Check sheet for the modelled part. Datum: model origin and axes. Units: mm. A direction names the side the tool comes from. Give positions to 0.01 mm unless a question says otherwise; leave off trailing zeros. Order: outer loops, then holes, each group sorted by start corner. A loop starts at its lowest first (then second) coordinate and runs counter-clockwise, first axis right, second up.
Autodesk Inventor part; units mm, degrees
ref_plane "Work Plane1" through (80, 0, 9.5) normal (0, 0, 1) x (1, 0, 0)
ref_plane "YZ Plane" through (0, 0, 0) normal (1, 0, 0) x (0, 1, 0)
ref_plane "XZ Plane" through (0, 0, 0) normal (0, 1, 0) x (-1, 0, 0)
sketch "Sketch1" plane through (0, 0, 0) normal (0, 0, 1) x (1, 0, 0)
  line L0 (0, 0) -> (115, 0)
  line L1 (115, 0) -> (115, 8.2)
  line L2 (115, 8.2) -> (-25, 8.2)
  line L3 (-25, 8.2) -> (-460, 8.2)
  line L4 (-460, 8.2) -> (-460, 0)
  line L5 (-460, 0) -> (0, 0)
  line L6 (-340, 8.2) -> (-340, 8.5)
  line L7 (-340, 8.5) -> (-390, 8.5)
  line L8 (-390, 8.5) -> (-390, 8.2)
  line L9 (15, 8.2) -> (15, 8.5)
  line L10 (15, 8.5) -> (-30, 8.5)
  line L11 (-30, 8.5) -> (-30, 8.2)
  line L12 (115, 8.2) -> (115, 9.5)
  line L13 (115, 9.5) -> (45, 9.5)
  line L14 (45, 9.5) -> (45, 8.2)
  line L15 (45, 9.5) -> (45, 10)
  line L16 (45, 10) -> (40, 10)
  line L17 (40, 10) -> (40, 8.2)
  line L18 (0, 8.5) -> (0, 7.5)
  line L19 (0, 7.5) -> (2, 7.5)
  line L20 (2, 7.5) -> (2, 8.5)
  line L21 (-460, 5) -> (-450, 5)
  line L22 (-450, 5) -> (-450, 8.2)
  dimension "d0" = 16.4
  dimension "d3" = 17
  dimension "d5" = 50
  dimension "d6" = 460
  dimension "d7" = 45
  dimension "d9" = 17
  dimension "d10" = 115
  dimension "d11" = 19
  dimension "d12" = 20
  dimension "d13" = 5
  dimension "d14" = 70
  dimension "d16" = 15
  dimension "d17" = 2
  dimension "d18" = 15
  dimension "d19" = 340
  dimension "d25" = 10
  dimension "d26" = 10
revolve "Revolution1" add sketch "Sketch1" angle 360 about axis through (0, 0, 0) along (1, 0, 0) contours L5 L4 L21 L22 L3 L2 L18 L19 L20 L1 L0 | L2 L14 L13 L12 | L2 L17 L16 L15 L14 | L2 L20 L10 L9 | L8 L7 L6 L3 | L2 L3 L11 L10 L18
ref_plane "Work Plane1" through (80, 0, 9.5) normal (0, 0, 1) x (1, 0, 0)
sketch "Sketch2" plane through (80, 0, 9.5) normal (0, 0, 1) x (1, 0, 0)
  line L0 (35, -9.5) -> (35, 9.5)
  line L1 (25, 0) -> (-25, 0) construction
  line L2 (25, 3) -> (-25, 3)
  line L3 (-25, -3) -> (25, -3)
  arc A0 (25, -3) -> (25, 3) centre (25, 0) ccw
  arc A1 (-25, 3) -> (-25, -3) centre (-25, 0) ccw
  point P0 (-80, 0)
  point P1 (0, 0)
  point P2 (35, 0)
  dimension "d20" = 6
  dimension "d21" = 50
  dimension "d22" = 35
extrude "Extrusion1" cut sketch "Sketch2" against normal blind 3
properties part number "shaft 2"
1) Section check A-A, the plane x = 71. Record the cut outline in (y, z), then the cut area to 3 significant figures.
Recorded:
outline: (-3, 6.5) - (-3, 9.01) arc R9.5 ccw (long way) to (3, 9.01) - (3, 6.5) - close
area: 266 mm2
2) Draft check along X on faces 5 (the face through (115, 0, 0)), 6 (the face through (-420.42, -1.07, -8.13)), 7 (the face through (2, 0, -8)). Enter one of: +X half, -X half, draft (parallel to the pull), parting line (faces both ways), or undercut.
Recorded:
face 5: +X half
face 6: draft
face 7: undercut
3) Material ranges on L1, parallel to X at y = 0.5, z = 6.75; L2, parallel to X at y = 3.5, z = 4.25; L3, parallel to X at y = 7.25, z = 3.25, recorded low to high.
Recorded:
L1: x = -450 to 52.04, 107.96 to 115
L2: x = -450 to 115
L3: x = -450 to 0, 2 to 115
4) Depth check by flat-ended pin: pin 1 Ø0.8 at (x, z) = (68.5, 7.5) entering from -Y; pin 2 Ø8 at (x, z) = (-84, -1) entering from +Y; pin 3 Ø4 at (x, z) = (-178, -5) entering from +Y. Enter the tip coordinate at first touch or a pass-through.
Recorded:
pin 1: stops at y = -6.31
pin 2: stops at y = 8.2
pin 3: stops at y = 7.63
5) Set-up check for faces 1 (the face through (42.46, -2.17, 9.76)), 2 (the face through (1.014, -7.493, 0.33)), 3 (the face through (-365.35, 4.57, -7.167)), 4 (the face through (45, 9, -4)): record each of +Z, -Z, +X, -X, +Y, -Y from which the full face is reachable in a straight line by a thin tool's end or side.
Recorded:
face 1: +X, -X
face 2: none
face 3: -X
face 4: +X
